Design review of the part built by this model. Coordinates are the model's own, in mm. Face numbers are marked on the shaded views. A direction names the side the tool comes from. Give positions to 0.01 mm unless a question says otherwise; leave off trailing zeros. Loops run counter-clockwise (first coordinate to the right, second up) from the corner with the lowest first, then second, coordinate; pieces in that order, holes last. Notation, with made-up numbers: M 4.5,78 L 45.5,78 A20 cw 45.5,104 Z; hole C 57,3.5 d8. An arc over 180 degrees is marked long. Use CSV: the item, a comma, the result in double quotes.
from build123d import *

# Parameters (mm, degrees)
F2_R     = 1.5875
F3_DEPTH = 6.35


with BuildPart() as f1:
    # F0 (on Front) → F1 (revolve)
    with BuildSketch(Plane.XZ):
        Polygon((0, 52.9984), (0, 0), (1.5875, 0), (1.5875, 15), (13.9954, 15), (13.9954, 52.9984), align=None)
    revolve(axis=Axis((0, 0, 34.635175), (0, 0, 1)))

    # F2 (on face) → F3 (cut)
    with BuildSketch(Plane(origin=(0, 0, 15), x_dir=(1, 0, 0), z_dir=(0, 0, -1))):
        with Locations((8.89, 0)):
            Circle(F2_R)
        with Locations((0, 8.89)):
            Circle(F2_R)
        with Locations((0, -8.89)):
            Circle(F2_R)
        with Locations((-8.89, 0)):
            Circle(F2_R)
    extrude(amount=-F3_DEPTH, mode=Mode.SUBTRACT)


solid = f1.part
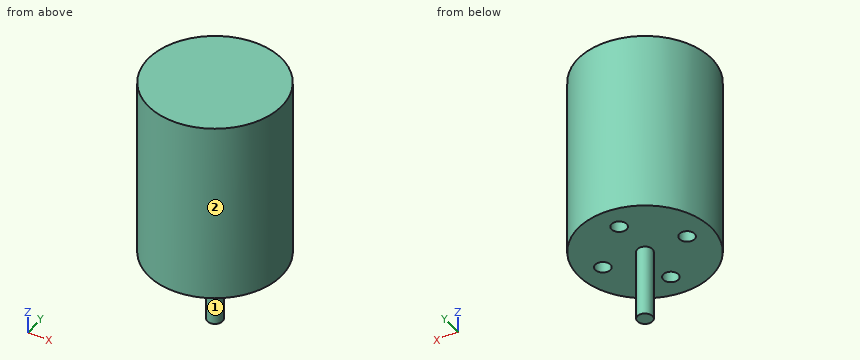
(1) We need section A-A on z = 18. State the section outline as (x, y) points (1 decimal).
A:
outline,"C 0,0 d28; hole C -8.9,0 d3.2; hole C 0,-8.9 d3.2; hole C 0,8.9 d3.2; hole C 8.9,0 d3.2"
(2) We need section B-B on x = 0. State the section outline as (y, z) points, then the cut area to 3 significant figures.
A:
outline,"M -14,15 L -10.48,15 L -10.48,21.35 L -7.3,21.35 L -7.3,15 L -1.59,15 L -1.59,0 L 1.59,0 L 1.59,15 L 7.3,15 L 7.3,21.35 L 10.48,21.35 L 10.48,15 L 14,15 L 14,53 L -14,53 Z"
area,"1,070 mm²"
(3) Clearance check with flat-ended pins moving along their axes: P1, Ø12, axis at x = 11, z = 43, coming from the +Y side; P2, Ø2.5, axis at x = 0.5, y = 8, coming from the -Z side; P3, Ø1.6, axis at x = -8.5, y = 0.5, coming from the -Z side. State where each tip first meets the part, or that it passes through.
A:
P1,"y = 13.07"
P2,"z = 15"
P3,"z = 21.35"
(4) We need section D-D on z = 11. State the section outline as (x, y) points (1 decimal), then the cut area to 3 significant figures.
A:
outline,"C 0,0 d3.2"
area,"7.92 mm²"
(5) Wall thickness on line 1 along Y through (x, z) = (0, 17.25); line 2 along Z through (x, y) = (-11.25, 7); line 3 along Z through (x, y) = (8.5, 0): over which ranges is each line inside the solid? List them lowest first. Write a range as [from, to].
A:
line 1,"[-14, -10.48], [-7.3, 7.3], [10.48, 14]"
line 2,"[15, 53]"
line 3,"[21.35, 53]"
(6) Machinability: for the marked faces 1 and 2, which of the approach directions +Z, -Z, +X, -X, +Y, -Y give a long, thin tool a straight path to every point of the face, cutting with its end or side? Answer none if there is none.
A:
face 1,"-Z"
face 2,"+Z, -Z"
